The model under review builds one solid part; all positions refer to its coordinate system, in mm. Face numbers are marked on the shaded views. Round coordinates to 2 decimals unless told otherwise and drop trailing zeros. Order: outer loops, then holes, each group sorted by start corner. A loop starts at its lowest first (then second) coordinate and runs counter-clockwise, first axis right, second up. Notation, with made-up numbers: M 80,64.25 L 94,64.25 A20 ccw 94,73.25 Z; hole C -32,70 d6. An arc over 180 degrees is marked long. One line per item, written item: value. Start each with the question number.
from build123d import *

# Parameters (mm, degrees)
F1_DEPTH  = 25.4
F2_T      = -5.08
F4_DEPTH  = 5.08
F6_DEPTH  = 5.08
F7_R      = 2.0955
F8_DEPTH  = 5.08
F9_R      = 3.175
F9_R_2    = 2.0955
F10_DEPTH = 2.54
F11_W     = 25.4
F11_H     = 12.7
F12_DEPTH = 5.08


# Not quite as in the source:
# - a shell that OpenCascade refuses in one call is made with other operations: the cavity is built on its own and cut out


with BuildPart() as f1:
    # F0 (on Front) → F1 (new body)
    with BuildSketch(Plane.XZ):
        with BuildLine():
            Line((43.9080937201, 75.5717812867), (-90.7119062799, 75.5717812867))
            ThreePointArc((-90.7119062799, 75.5717812867), (-95.2020343405, 73.7119093473), (-97.0619062799, 69.2217812867))
            Line((-97.0619062799, 69.2217812867), (-97.0619062799, 5.7217812867))
            ThreePointArc((-97.0619062799, 5.7217812867), (-95.2020343405, 1.2316532262), (-90.7119062799, -0.6282187133))
            Line((-90.7119062799, -0.6282187133), (43.9080937201, -0.6282187133))
            ThreePointArc((43.9080937201, -0.6282187133), (48.3982217806, 1.2316532262), (50.2580937201, 5.7217812867))
            Line((50.2580937201, 5.7217812867), (50.2580937201, 69.2217812867))
            ThreePointArc((50.2580937201, 69.2217812867), (48.3982217806, 73.7119093473), (43.9080937201, 75.5717812867))
        make_face()
    extrude(amount=F1_DEPTH)

    # F2: a shell. OpenCascade refuses it in one call, so the cavity is built on its own and cut out:
    # the body offset inwards by the wall thickness, plus a prism from it out through each open face.
    f2_core = offset(f1.part, amount=F2_T, mode=Mode.PRIVATE)
    f2_exits = [f2_core.faces().sort_by_distance(p)[0] for p in [
        (-23.401906, -12.7, 70.491781),
    ]]
    add(f2_core, mode=Mode.SUBTRACT)
    extrude(f2_exits, amount=-F2_T, mode=Mode.SUBTRACT)

    # F3 (on face) → F4 (cut)
    with BuildSketch(Plane.XZ.offset(25.4)):
        with BuildLine():
            Line((35.0180937201, 75.5717812867), (-81.8219062799, 75.5717812867))
            Line((-81.8219062799, 75.5717812867), (-81.8219062799, 17.1517812867))
            ThreePointArc((-81.8219062799, 17.1517812867), (-79.9620343405, 12.6616532262), (-75.4719062799, 10.8017812867))
            Line((-75.4719062799, 10.8017812867), (28.6680937201, 10.8017812867))
            ThreePointArc((28.6680937201, 10.8017812867), (33.1582217806, 12.6616532262), (35.0180937201, 17.1517812867))
            Line((35.0180937201, 17.1517812867), (35.0180937201, 75.5717812867))
        make_face()
    extrude(amount=-F4_DEPTH, mode=Mode.SUBTRACT)

    # F5 (on face) → F6 (cut)
    with BuildSketch(Plane(origin=(0, 0, 0), x_dir=(-1, 0, 0), z_dir=(0, 1, 0))):
        with BuildLine():
            Line((-26.1280937201, 62.8717812867), (-31.2080937201, 62.8717812867))
            ThreePointArc((-31.2080937201, 62.8717812867), (-35.6982217806, 61.0119093473), (-37.5580937201, 56.5217812867))
            Line((-37.5580937201, 56.5217812867), (-37.5580937201, 18.4217812867))
            ThreePointArc((-37.5580937201, 18.4217812867), (-35.6982217806, 13.9316532262), (-31.2080937201, 12.0717812867))
            Line((-31.2080937201, 12.0717812867), (-26.1280937201, 12.0717812867))
            ThreePointArc((-26.1280937201, 12.0717812867), (-21.6379656595, 13.9316532262), (-19.7780937201, 18.4217812867))
            Line((-19.7780937201, 18.4217812867), (-19.7780937201, 56.5217812867))
            ThreePointArc((-19.7780937201, 56.5217812867), (-21.6379656595, 61.0119093473), (-26.1280937201, 62.8717812867))
        make_face()
        with BuildLine():
            Line((78.0119062799, 62.8717812867), (73.519602201, 62.8717812867))
            ThreePointArc((73.519602201, 62.8717812867), (69.0294741405, 61.0119093473), (67.169602201, 56.5217812867))
            Line((67.169602201, 56.5217812867), (67.169602201, 18.4217812867))
            ThreePointArc((67.169602201, 18.4217812867), (69.0294741405, 13.9316532262), (73.519602201, 12.0717812867))
            Line((73.519602201, 12.0717812867), (78.0119062799, 12.0717812867))
            ThreePointArc((78.0119062799, 12.0717812867), (82.5020343405, 13.9316532262), (84.3619062799, 18.4217812867))
            Line((84.3619062799, 18.4217812867), (84.3619062799, 56.5217812867))
            ThreePointArc((84.3619062799, 56.5217812867), (82.5020343405, 61.0119093473), (78.0119062799, 62.8717812867))
        make_face()
    extrude(amount=-F6_DEPTH, mode=Mode.SUBTRACT)

    # F7 (on face) → F8 (cut)
    with BuildSketch(Plane.XZ.offset(5.08)):
        with Locations((-23.4019062799, 45.4727812867)):
            Circle(F7_R)
        with Locations((-31.4029062799, 37.4717812867)):
            Circle(F7_R)
        with Locations((-23.4019062799, 29.4707812867)):
            Circle(F7_R)
        with Locations((-15.4009062799, 37.4717812867)):
            Circle(F7_R)
    extrude(amount=-F8_DEPTH, mode=Mode.SUBTRACT)

    # F9 (on face) → F10 (cut)
    with BuildSketch(Plane.XZ.offset(5.08)):
        with Locations((-31.4029062799, 37.4717812867)):
            Circle(F9_R)
        with Locations((-31.4029062799, 37.4717812867)):
            Circle(F9_R_2, mode=Mode.SUBTRACT)
        with Locations((-23.4019062799, 45.4727812867)):
            Circle(F9_R)
        with Locations((-23.4019062799, 45.4727812867)):
            Circle(F9_R_2, mode=Mode.SUBTRACT)
        with Locations((-15.4009062799, 37.4717812867)):
            Circle(F9_R)
        with Locations((-15.4009062799, 37.4717812867)):
            Circle(F9_R_2, mode=Mode.SUBTRACT)
        with Locations((-23.4019062799, 29.4707812867)):
            Circle(F9_R)
        with Locations((-23.4019062799, 29.4707812867)):
            Circle(F9_R_2, mode=Mode.SUBTRACT)
    extrude(amount=-F10_DEPTH, mode=Mode.SUBTRACT)

    # F11 (on face) → F12 (cut)
    with BuildSketch(Plane(origin=(0, 0, -0.6282187133), x_dir=(1, 0, 0), z_dir=(0, 0, -1))):
        with Locations((-52.6119062799, 13.97)):
            Rectangle(F11_W, F11_H)
        with Locations((5.8080937201, 13.97)):
            Rectangle(F11_W, F11_H)
    extrude(amount=-F12_DEPTH, mode=Mode.SUBTRACT)


solid = f1.part
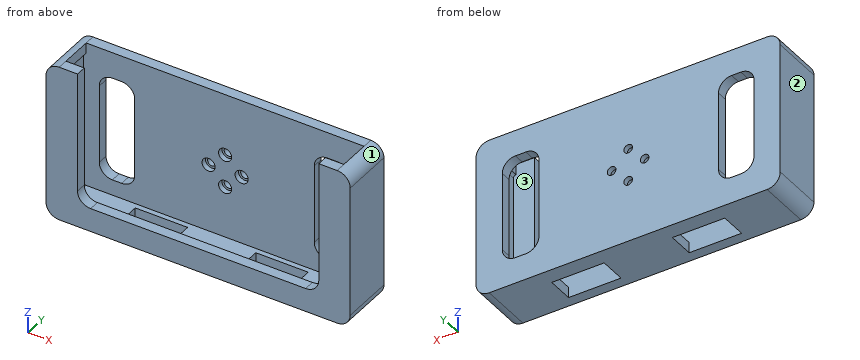
Item 1: Wall thickness on L1, parallel to X at y = -2, z = 25.5; L2, parallel to Y at x = -30, z = 5.5; L3, parallel to X at y = -22.25, z = 24.5: over which ranges is each line inside the solid? List them lowest first.
Item 2: Clearance check with flat-ended pins moving along their axes: P1, Ø2.5, axis at y = -16.5, z = 1.5, coming from the +X side; P2, Ø4, axis at y = -15.5, z = 3, coming from the -X side; P3, Ø8.5, axis at x = -15.4, z = 37.47, coming from the -Y side. State where each tip first meets the part, or that it passes through.
Item 3: Consider section B-B, the plane z = 23. Give the boundary of the cut face in (x, y), then the cut area to 3 significant figures.
Item 4: Consider section A-A, the plane y = -12.5. Give the boundary of the cut face in (x, z), then the cut area to 3 significant figures.
Item 5: Consider section C-C, the plane x = 24. Give the boundary of the cut face in (y, z), then the cut area to 3 significant figures.
Item 6: The part is to be moulded in two halves that separate along X. For the marked faces 1, 2 and 3, say which applies: pulls with the +X half, pulls with the -X half, needs draft (parallel to the pull), parting line crosses it, or undercut.
Computed:
1. L1: x = -97.06 to -84.36, -67.17 to 19.78, 37.56 to 50.26
1. L2: y = -25.4 to -20.32, -5.08 to 0
1. L3: x = -97.06 to -81.82, 35.02 to 50.26
2. P1: stops at x = 49.52
2. P2: stops at x = -97.02
2. P3: stops at y = -5.08
3. outline: M -97.06,-25.4 L -81.82,-25.4 L -81.82,-20.32 L -91.98,-20.32 L -91.98,-5.08 L -84.36,-5.08 L -84.36,0 L -97.06,0 Z; M -67.17,-5.08 L 19.78,-5.08 L 19.78,0 L -67.17,0 Z; M 35.02,-25.4 L 50.26,-25.4 L 50.26,0 L 37.56,0 L 37.56,-5.08 L 45.18,-5.08 L 45.18,-20.32 L 35.02,-20.32 Z
3. area: 880 mm^2
4. outline: M -97.06,5.72 A6.35 ccw -90.71,-0.63 L -65.31,-0.63 L -65.31,4.45 L -90.71,4.45 A1.27 cw -91.98,5.72 L -91.98,69.22 A1.27 cw -90.71,70.49 L -90.71,75.57 A6.35 ccw -97.06,69.22 Z; M -39.91,-0.63 L -6.89,-0.63 L -6.89,4.45 L -39.91,4.45 Z; M 18.51,-0.63 L 43.91,-0.63 A6.35 ccw 50.26,5.72 L 50.26,69.22 A6.35 ccw 43.91,75.57 L 43.91,70.49 A1.27 cw 45.18,69.22 L 45.18,5.72 A1.27 cw 43.91,4.45 L 18.51,4.45 Z
4. area: 1,190 mm^2
5. outline: M -25.4,-0.63 L 0,-0.63 L 0,12.44 L -5.08,12.44 L -5.08,4.45 L -20.32,4.45 L -20.32,10.8 L -25.4,10.8 Z; M -5.08,62.5 L 0,62.5 L 0,75.57 L -5.08,75.57 Z
5. area: 268 mm^2
6. face 1: pulls with the +X half
6. face 2: pulls with the -X half
6. face 3: undercut
